Part model, mm, in its own coordinate system. A direction names the side the tool comes from. Round coordinates to 2 decimals unless told otherwise and drop trailing zeros. Loops run counter-clockwise (first coordinate to the right, second up) from the corner with the lowest first, then second, coordinate; pieces in that order, holes last.
(1) Cut at A-A on z = -15. List the corners of the cut face in (x, y).
(2) Cut at B-B on y = 5. List the corners of the cut face in (x, z).
(3) Probe probe 1 along Y at (x, z) = (-19, -25); probe 2 along Y at (x, z) = (-9, -24); probe 3 along Y at (x, z) = (2.5, 3.35). List the from-to ranges inside material, lowest first.
(4) Mould opens along Z. For faces 5 (the face through (10, 15, 2)), 6 (the face through (-24, 5, -27.61)) say: +Z half, -Z half, draft (parallel to the pull), parting line (faces both ways), or undercut.
(5) Tool access for faces 1 (the face through (-23.521, 25.942, -22.495)), 2 (the face through (-25, 15, -15)), 3 (the face through (-15.5, 15, -26)), 4 (the face through (-6.52, 3.31, -23.16)): list every direction of +Z, -Z, +X, -X, +Y, -Y with a clear straight run to the whole face (end or side of a thin tool).
(6) Flat gauge pins, fed straight in: pin 1 (6.5 mm diameter, centred on y = 25, z = -24, fed in from -X); pin 2 (15 mm diameter, centred on y = 8.5, z = -18.5, fed in from +X); pin 3 (2.5 mm diameter, centred on y = 5, z = -25, fed in from +X); pin 4 (3.5 mm diameter, centred on y = 25, z = -25, fed in from -X). Where does each tip first touch, or does it go through?
(7) Cut at C-C on x = 2.5. List the corners of the cut face in (y, z).
(8) Cut at D-D on x = -11.5. List the corners of the cut face in (y, z).
Autodesk Inventor part; units mm, degrees
ref_plane "YZ Plane" through (0, 0, 0) normal (1, 0, 0) x (0, 1, 0)
ref_plane "XZ Plane" through (0, 0, 0) normal (0, 1, 0) x (-1, 0, 0)
ref_plane "XY Plane" through (0, 0, 0) normal (0, 0, 1) x (1, 0, 0)
sketch "Sketch1" plane through (0, 0, 0) normal (0, 1, 0) x (-1, 0, 0)
  line L0 (5, 0) -> (25, 0)
  arc A0 (15.5, -21.4807) -> (14.5, -21.4807) centre (15, -15) ccw
  line L1 (14.5, -21.4807) -> (14.5, -30)
  line L2 (15.5, -30) -> (15.5, -21.4807)
  line L3 (14.5, -20.3939) -> (15.5, -30) construction
  line L4 (14.5, -30) -> (15.386, -21.4885) construction
  line L5 (25, -30) -> (15.5, -30)
  line L6 (14.5, -30) -> (5, -30)
  line L7 (25, 0) -> (25, -30)
  line L8 (5, 0) -> (5, -30)
  line L9 (25, 0) -> (40, 0)
  line L10 (40, 0) -> (40, 5)
  line L11 (5, 0) -> (-10, 0)
  line L12 (-10, 0) -> (-10, 5)
  line L13 (-10, 5) -> (40, 5)
  point P0 (0, 0)
  point P1 (15, -25.1969)
  dimension "d2" = 13
  dimension "d26" = 15
  dimension "d28" = 15
extrude "Extrusion1" add sketch "Sketch1" along normal blind 30
hole "Hole1" at (-5, 25, -25) direction (-1, 0, 0) diameter 3 end through all counterbore diameter 5 counterbore depth 3
hole "Hole2" at (-5, 5, -25) direction (-1, 0, 0) diameter 3 end through all counterbore diameter 5 counterbore depth 3
sketch "Sketch2" plane through (-25, 0, -30) normal (-1, 0, 0) x (0, 0, 1)
  circle A0 centre (5, 25) radius 1.5
  line L0 (3.9359, 27.9014) -> (6.9806, 27.3722)
  line L1 (6.9806, 27.3722) -> (8.0447, 24.4708)
  line L2 (8.0447, 24.4708) -> (6.0641, 22.0986)
  line L3 (6.0641, 22.0986) -> (3.0194, 22.6278)
  line L4 (3.0194, 22.6278) -> (1.9553, 25.5292)
  line L5 (1.9553, 25.5292) -> (3.9359, 27.9014)
  circle A1 centre (5, 5) radius 1.5
  line L6 (5, 8.0137) -> (7.61, 6.5069)
  line L7 (7.61, 6.5069) -> (7.61, 3.4931)
  line L8 (7.61, 3.4931) -> (5, 1.9863)
  line L9 (5, 1.9863) -> (2.39, 3.4931)
  line L10 (2.39, 3.4931) -> (2.39, 6.5069)
  line L11 (2.39, 6.5069) -> (5, 8.0137)
  point P0 (30, 0)
extrude "Extrusion2" cut sketch "Sketch2" against normal blind 3
hole "Hole3" at (-32.5, 15, 0) direction (0, 0, 1) diameter 6 end through all
hole "Hole4" at (2.5, 15, 0) direction (0, 0, 1) diameter 6 end through all
properties part number "WaterPumpHolder"
Final values:
1. outline: (-25, 0) - (-21.5, 0) - (-21.5, 30) - (-25, 30) - close; (-8.5, 0) - (-5, 0) - (-5, 30) - (-8.5, 30) - close
2. outline: (-40, 0) - (-25, 0) - (-25, -22.39) - (-22, -22.39) - (-22, -23.5) - (-15.5, -23.5) - (-15.5, -21.48) arc R6.5 cw (long way) to (-14.5, -21.48) - (-14.5, -23.5) - (-8, -23.5) - (-8, -22.5) - (-5, -22.5) - (-5, 0) - (10, 0) - (10, 5) - (-40, 5) - close; (-25, -30) - (-15.5, -30) - (-15.5, -26.5) - (-22, -26.5) - (-22, -27.61) - (-25, -27.61) - close; (-14.5, -30) - (-5, -30) - (-5, -27.5) - (-8, -27.5) - (-8, -26.5) - (-14.5, -26.5) - close
3. probe 1: y = 0 to 3.5, 6.5 to 23.5, 26.5 to 30
3. probe 2: y = 0 to 3.88, 6.12 to 23.88, 26.12 to 30
3. probe 3: y = 0 to 12, 18 to 30
4. face 5: draft
4. face 6: undercut
5. face 1: -X
5. face 2: -Z, -X, +Y, -Y
5. face 3: -Z, +Y, -Y
5. face 4: +X
6. pin 1: stops at x = -25
6. pin 2: stops at x = -5
6. pin 3: passes through
6. pin 4: stops at x = -22
7. outline: (0, 0) - (12, 0) - (12, 5) - (0, 5) - close; (18, 0) - (30, 0) - (30, 5) - (18, 5) - close
8. outline: (0, -30) - (30, -30) - (30, -20.48) - (0, -20.48) - close; (0, -9.52) - (30, -9.52) - (30, 5) - (0, 5) - close; hole circle Ø3 at (5, -25); hole circle Ø3 at (25, -25)
